```python
from build123d import *

# Parameters (mm, degrees)
CROQUIS1_W                     = 66.04
CROQUIS1_H                     = 83.058
SALIENTE_EXTRUIR1_DEPTH        = 1
TALADRO_DE_MARGEN_PARA_M2_51_D = 2.7
CROQUIS9_R                     = 0.45
SALIENTE_EXTRUIR2_DEPTH        = 17


with BuildPart() as part:
    # Croquis1 → Saliente-Extruir1 (new body)
    with BuildSketch(Plane.XY):
        with Locations((33.02, 41.529)):
            Rectangle(CROQUIS1_W, CROQUIS1_H)
    extrude(amount=SALIENTE_EXTRUIR1_DEPTH)

    # Taladro de margen para M2.51 (through all)
    with Locations(Plane(origin=(5.51942, 69.37502, 1), x_dir=(1, 0, 0), z_dir=(0, 0, 1))):
        with Locations((0, 0), (55.00116, 0), (3.54838, -63.00216), (51.45278, -63.00216)):
            Hole(TALADRO_DE_MARGEN_PARA_M2_51_D / 2)

    # Croquis9 → Saliente-Extruir2 (add)
    with BuildSketch(Plane.XY.offset(1)):
        with Locations((57.15, 57.658)):
            Circle(CROQUIS9_R)
        with Locations((57.15, 55.118)):
            Circle(CROQUIS9_R)
        with Locations((57.15, 52.578)):
            Circle(CROQUIS9_R)
        with Locations((57.15, 50.038)):
            Circle(CROQUIS9_R)
        with Locations((57.15, 44.958)):
            Circle(CROQUIS9_R)
        with Locations((57.15, 39.878)):
            Circle(CROQUIS9_R)
        with Locations((57.15, 37.338)):
            Circle(CROQUIS9_R)
        with Locations((57.15, 47.498)):
            Circle(CROQUIS9_R)
        with Locations((57.15, 42.418)):
            Circle(CROQUIS9_R)
        with Locations((57.15, 34.798)):
            Circle(CROQUIS9_R)
        with Locations((57.15, 30.734)):
            Circle(CROQUIS9_R)
        with Locations((57.15, 28.194)):
            Circle(CROQUIS9_R)
        with Locations((57.15, 25.654)):
            Circle(CROQUIS9_R)
        with Locations((57.15, 20.574)):
            Circle(CROQUIS9_R)
        with Locations((57.15, 23.114)):
            Circle(CROQUIS9_R)
        with Locations((57.15, 15.494)):
            Circle(CROQUIS9_R)
        with Locations((57.15, 18.034)):
            Circle(CROQUIS9_R)
        with Locations((8.89, 23.114)):
            Circle(CROQUIS9_R)
        with Locations((8.89, 20.574)):
            Circle(CROQUIS9_R)
        with Locations((8.89, 18.034)):
            Circle(CROQUIS9_R)
        with Locations((8.89, 15.494)):
            Circle(CROQUIS9_R)
        with Locations((8.89, 30.734)):
            Circle(CROQUIS9_R)
        with Locations((57.15, 12.954)):
            Circle(CROQUIS9_R)
        with Locations((8.89, 25.654)):
            Circle(CROQUIS9_R)
        with Locations((8.89, 12.954)):
            Circle(CROQUIS9_R)
        with Locations((8.89, 48.514)):
            Circle(CROQUIS9_R)
        with Locations((8.89, 45.974)):
            Circle(CROQUIS9_R)
        with Locations((8.89, 43.434)):
            Circle(CROQUIS9_R)
        with Locations((8.89, 38.354)):
            Circle(CROQUIS9_R)
        with Locations((8.89, 40.894)):
            Circle(CROQUIS9_R)
        with Locations((8.89, 33.274)):
            Circle(CROQUIS9_R)
        with Locations((8.89, 35.814)):
            Circle(CROQUIS9_R)
    extrude(amount=-SALIENTE_EXTRUIR2_DEPTH)


solid = part.part
```
Work out the finished part from the listing and answer in its coordinate system (mm). Give positions to 0.01 mm unless a question says otherwise; leave off trailing zeros. Write each loop counter-clockwise with the first axis right and the second up, starting at its lowest first coordinate (ties: lowest second). Pieces come first, ordered by that corner, then holes. Notation, with made-up numbers: (74, 24.5) -> (129, 24.5) arc R30 ccw to (129, 55.5) -> close; hole circle Ø5 at (26, 85.5). An arc over 180 degrees is marked (long way). Write each question's results on one line, items separated by ' | '.
1. Find section A-A on z = -2. Give the number of separate pieces and of enclosed holes in the cut face, and give its area (3 significant figures).
Data:
separate pieces: 32 | enclosed holes: 0 | area: 20.4 mm^2
2. Each of these flat-tipped pins is pushed along its axis until it touches: pin 1 Ø1.6 at (x, y) = (5.52, 69.38) entering from -Z; pin 2 Ø2 at (y, z) = (37, -11.5) entering from +X; pin 3 Ø2 at (y, z) = (16, -1.5) entering from -X; pin 4 Ø8 at (x, z) = (7, -13) entering from -Y. Where does it stop, or does it pass through?
Data:
pin 1: through | pin 2: x = 57.6 | pin 3: x = 8.44 | pin 4: y = 12.5
3. Find section B-B on x = 34. Determine the outline of the cut face in (y, z).
Data:
outline: (0, 0) -> (83.06, 0) -> (83.06, 1) -> (0, 1) -> close
4. Determine the mould class of faces 1 (the flat face through (33, 42, 1)), 2 (the cylindrical face through (61.516, 70.287, 0.493)), 3 (the cylindrical face through (10.416, 6.432, 0.493)) for opening direction X: +X half, -X half, draft (parallel to the pull), parting line (faces both ways), or undercut.
Data:
face 1: draft | face 2: undercut | face 3: undercut
5. Straight lines are drawn through the part: L1, parallel to Z at x = 59.5, y = 14; L2, parallel to X at y = 52.5, z = -11; L3, parallel to X at y = 31, z = -6.5. For each, find the intervals that lie inside material, in ascending order.
Data:
L1: 0 to 1 | L2: 56.71 to 57.59 | L3: 8.53 to 9.25, 56.79 to 57.51
